Study the drawing (mm; zero at the part's minimum x, y, z) and answer. A direction names the side the tool comes from. Give positions to 0.01 mm unless a question says otherwise; leave off trailing zeros. Order: outer loops, then holes, each group sorted by start corner. A loop starts at its lowest first (then second) coordinate and runs counter-clockwise, first axis right, second up.
Item 1: A cutting plane is placed at C-C (y = 2). Write down the section's boundary in (x, z), plus the area to 3 significant figures.
Item 2: Which of the six approach directions +Z, -Z, +X, -X, +Y, -Y give full straight-line access (tool end or side, diameter ignored) to the marked faces 1 and 2?
Item 3: A cutting plane is placed at B-B (x = 18). Write down the section's boundary in (y, z).
Item 4: Find the intervals of material crossed by line 1 along X through (y, z) = (5.25, 4.65); line 2 along Y through (x, z) = (50.5, 2.8); line 3 along X through (y, z) = (1.75, 2.55), in increasing order.
Item 5: A cutting plane is placed at A-A (z = 0.65). Write down the section's boundary in (x, y), plus the area to 3 significant figures.
Item 6: Given pin 1 Ø1.5 at (x, z) = (9, 2.5) entering from -Y; pin 2 Ø1.5 at (x, z) = (12, 3) entering from -Y, each flat-ended and moving along its own axis, determine where each tip first touches the part or whether it passes through.
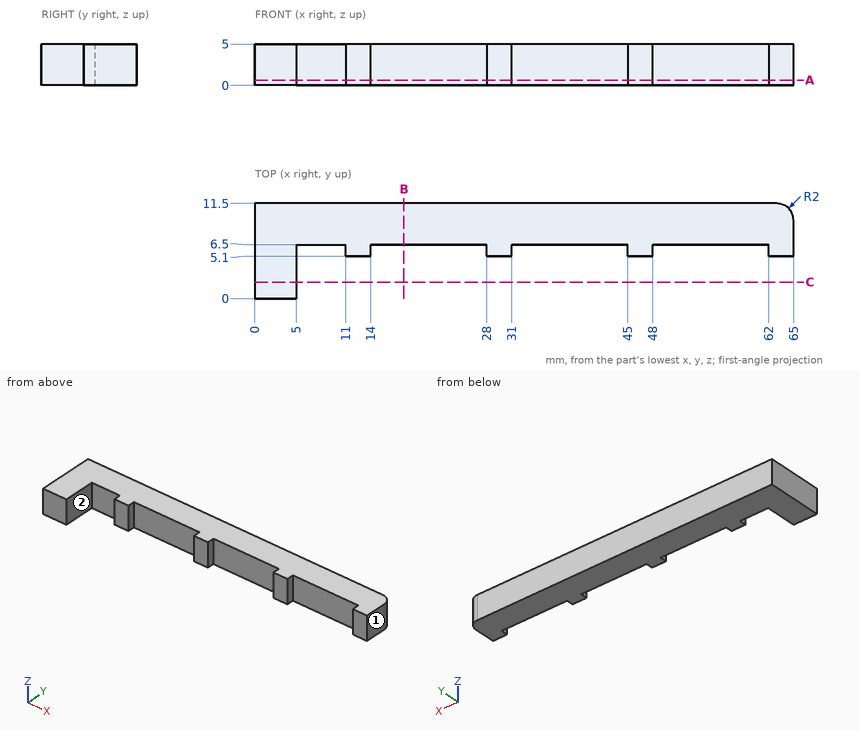
Response values:
1. outline: (0, 0) - (5, 0) - (5, 5) - (0, 5) - close
1. area: 25.0 mm2
2. face 1: +Z, -Z, +X, +Y, -Y
2. face 2: +Z, -Z, -Y
3. outline: (6.5, 0) - (11.5, 0) - (11.5, 5) - (6.5, 5) - close
4. line 1: x = 0 to 5, 11 to 14, 28 to 31, 45 to 48, 62 to 65
4. line 2: y = 6.5 to 11.5
4. line 3: x = 0 to 5
5. outline: (0, 0) - (5, 0) - (5, 6.5) - (11, 6.5) - (11, 5.1) - (14, 5.1) - (14, 6.5) - (28, 6.5) - (28, 5.1) - (31, 5.1) - (31, 6.5) - (45, 6.5) - (45, 5.1) - (48, 5.1) - (48, 6.5) - (62, 6.5) - (62, 5.1) - (65, 5.1) - (65, 9.5) arc R2 ccw to (63, 11.5) - (0, 11.5) - close
5. area: 373 mm2
6. pin 1: stops at y = 6.5
6. pin 2: stops at y = 5.1
